Input: part model. Units: mm. Frame: model coordinates. Round coordinates to 2 decimals unless told otherwise and drop trailing zeros. Write each loop counter-clockwise with the first axis right and the second up, starting at its lowest first coordinate (ties: lowest second). Pieces come first, ordered by that corner, then holes. Notation, with made-up numbers: M 46,49.5 L 63,49.5 A26 ccw 63,70.5 Z; hole C 57.5,-20 d11. An arc over 180 degrees is marked long. Answer as CSV lines item,"result". Start each with the question number.
```python
from build123d import *

# Parameters (mm, degrees)
SKETCH1_R           = 2.413
BOSS_EXTRUDE1_DEPTH = 4.7625


with BuildPart() as part:
    # Sketch1 → Boss-Extrude1 (new body)
    with BuildSketch(Plane.XY):
        Polygon((101.6, 38.1), (50.8, 101.6), (0, 101.6), (0, 0), (101.6, 0), align=None)
        with Locations(Location((25.4, 19.05, 0), (0, 0, 180))):
            Circle(SKETCH1_R, mode=Mode.SUBTRACT)
        with Locations(Location((63.5, 19.05, 0), (0, 0, 180))):
            Circle(SKETCH1_R, mode=Mode.SUBTRACT)
        with Locations(Location((88.9, 19.05, 0), (0, 0, 180))):
            Circle(SKETCH1_R, mode=Mode.SUBTRACT)
        with Locations(Location((25.4, 57.15, 0), (0, 0, 180))):
            Circle(SKETCH1_R, mode=Mode.SUBTRACT)
        with Locations(Location((25.4, 88.9, 0), (0, 0, 180))):
            Circle(SKETCH1_R, mode=Mode.SUBTRACT)
    extrude(amount=BOSS_EXTRUDE1_DEPTH)


solid = part.part
```
Item 1: Cut plane B-B, the plane z = 0.75. Return loops of the section in (x, y), plus the area to 3 significant figures.
Item 2: Line query: line 1 (X direction, y = 19.05, z = 2.3); line 2 (Y direction, x = 25.4, z = 1.8); line 3 (Y direction, x = 88.9, z = 1.65) (3 decimals). Output: solid intervals per line, ascending. Write a range as [from, to].
Item 3: Cut plane C-C, the plane y = 57.15. Return loops of the section in (x, z), plus the area to 3 significant figures.
Item 4: Cut plane A-A, the plane x = 25.4. Return loops of the section in (y, z), plus the area to 3 significant figures.
Item 5: Cut plane D-D, the plane y = 19.05. Return loops of the section in (x, z).
Item 6: Pin query (flat end, axial travel): pin 1 Ø4.5 at (x, y) = (25.4, 57.15) entering from -Z. Return the tip coordinate at first contact, or that it passes through.
Item 7: Draft query along X for faces 1 (the face through (27.315, 58.618, 2.348)), 2 (the face through (76.556, 69.406, 2.348)), 3 (the face through (26, 101.6, 2)), 4 (the face through (86.67, 19.97, 2.35)). Return one class per face: +X half, -X half, draft (parallel to the pull), parting line (faces both ways), or undercut.
Results list:
1,outline,"M 0,0 L 101.6,0 L 101.6,38.1 L 50.8,101.6 L 0,101.6 Z; hole C 25.4,19.05 d4.83; hole C 25.4,57.15 d4.83; hole C 25.4,88.9 d4.83; hole C 63.5,19.05 d4.83; hole C 88.9,19.05 d4.83"
1,area,"8,620 mm²"
2,line 1,"[0, 22.99], [27.81, 61.09], [65.91, 86.49], [91.31, 101.6]"
2,line 2,"[0, 16.64], [21.46, 54.74], [59.56, 86.49], [91.31, 101.6]"
2,line 3,"[0, 16.637], [21.463, 53.975]"
3,outline,"M 0,0 L 22.99,0 L 22.99,4.76 L 0,4.76 Z; M 27.81,0 L 86.36,0 L 86.36,4.76 L 27.81,4.76 Z"
3,area,"388 mm²"
4,outline,"M 0,0 L 16.64,0 L 16.64,4.76 L 0,4.76 Z; M 21.46,0 L 54.74,0 L 54.74,4.76 L 21.46,4.76 Z; M 59.56,0 L 86.49,0 L 86.49,4.76 L 59.56,4.76 Z; M 91.31,0 L 101.6,0 L 101.6,4.76 L 91.31,4.76 Z"
4,area,"415 mm²"
5,outline,"M 0,0 L 22.99,0 L 22.99,4.76 L 0,4.76 Z; M 27.81,0 L 61.09,0 L 61.09,4.76 L 27.81,4.76 Z; M 65.91,0 L 86.49,0 L 86.49,4.76 L 65.91,4.76 Z; M 91.31,0 L 101.6,0 L 101.6,4.76 L 91.31,4.76 Z"
6,pin 1,"through"
7,face 1,"undercut"
7,face 2,"+X half"
7,face 3,"draft"
7,face 4,"undercut"
